```python
from build123d import *

# Parameters (mm, degrees)
SKETCH_1_W          = 45
SKETCH_1_H          = 70
SKETCH_1_R          = 2.25
SKETCH_1_R_2        = 2.5
SKETCH_1_R_3        = 1.75
SKETCH_1_R_4        = 0.9
SKETCH_1_R_5        = 0.75
EXTRUDE_1_DEPTH     = 1.5
SKETCH_2_R          = 0.6
CUT_EXTRUDE_1_DEPTH = 1.5


with BuildPart() as part:
    # Эскиз1 → Вытянуть1 (new body)
    with BuildSketch(Plane.XY):
        Rectangle(SKETCH_1_W, SKETCH_1_H)
        with Locations((-17.5, 30)):
            Circle(SKETCH_1_R, mode=Mode.SUBTRACT)
        with Locations(Location((17.5, 30, 0), (0, 0, 180))):
            Circle(SKETCH_1_R, mode=Mode.SUBTRACT)
        with Locations((17.5, -30)):
            Circle(SKETCH_1_R, mode=Mode.SUBTRACT)
        with Locations(Location((-17.5, -30, 0), (0, 0, 180))):
            Circle(SKETCH_1_R, mode=Mode.SUBTRACT)
        with Locations((0, -3)):
            Circle(SKETCH_1_R_2, mode=Mode.SUBTRACT)
        with Locations((-10.5, 7.5)):
            Circle(SKETCH_1_R_3, mode=Mode.SUBTRACT)
        with Locations((10.5, -13.5)):
            Circle(SKETCH_1_R_3, mode=Mode.SUBTRACT)
        with Locations((-5, 30)):
            Circle(SKETCH_1_R_4, mode=Mode.SUBTRACT)
        with Locations((0, 30)):
            Circle(SKETCH_1_R_4, mode=Mode.SUBTRACT)
        with Locations((5, 30)):
            Circle(SKETCH_1_R_4, mode=Mode.SUBTRACT)
        with Locations((-2.5, -30)):
            Circle(SKETCH_1_R_4, mode=Mode.SUBTRACT)
        with Locations((2.5, -30)):
            Circle(SKETCH_1_R_4, mode=Mode.SUBTRACT)
        with Locations((-4.5, -16.5)):
            Circle(SKETCH_1_R_5, mode=Mode.SUBTRACT)
        with Locations((-4.5, 10.5)):
            Circle(SKETCH_1_R_5, mode=Mode.SUBTRACT)
        with Locations(Location((4.5, -16.5, 0), (0, 0, 180))):
            Circle(SKETCH_1_R_5, mode=Mode.SUBTRACT)
        with Locations(Location((4.5, 10.5, 0), (0, 0, 180))):
            Circle(SKETCH_1_R_5, mode=Mode.SUBTRACT)
    extrude(amount=EXTRUDE_1_DEPTH)

    # Эскиз2 → Вырез-Вытянуть1 (cut)
    with BuildSketch(Plane.XY.offset(1.5)):
        with Locations((-17.5, -20.5)):
            Circle(SKETCH_2_R)
        with Locations((-17.5, 2.5)):
            Circle(SKETCH_2_R)
        with Locations(Location((17.5, 2.5, 0), (0, 0, 180))):
            Circle(SKETCH_2_R)
        with Locations(Location((17.5, -20.5, 0), (0, 0, 180))):
            Circle(SKETCH_2_R)
        with Locations((-7.5, -21.5)):
            Circle(SKETCH_2_R)
        with Locations((7.5, -21.5)):
            Circle(SKETCH_2_R)
        with Locations((-7.5, 15)):
            Circle(SKETCH_2_R)
        with Locations((7.5, 15)):
            Circle(SKETCH_2_R)
        with Locations((-10, 21.75)):
            Circle(SKETCH_2_R)
        with Locations(Location((10, 21.75, 0), (0, 0, 180))):
            Circle(SKETCH_2_R)
    extrude(amount=-CUT_EXTRUDE_1_DEPTH, mode=Mode.SUBTRACT)


solid = part.part
```
Geometry: final body of the model. Coordinates: model frame, mm. Round coordinates to 2 decimals unless told otherwise and drop trailing zeros. Write each loop counter-clockwise with the first axis right and the second up, starting at its lowest first coordinate (ties: lowest second). Pieces come first, ordered by that corner, then holes. Notation, with made-up numbers: M -22.75,39 L -2.75,39 A19 ccw -2.75,60 Z; hole C 50.25,-8 d9. An arc over 180 degrees is marked long. Answer in a Markdown table with one row per item. Add a question column.
(1) Ray query, L1, parallel to Y at x = 0, z = 0.45; L2, parallel to Y at x = 17.5, z = 0.45; L3, parallel to Y at x = -8, z = 1.25. Return the intervals inside material, ascending.
(2) Cut plane C-C, the plane x = 16. Return the cut outline in (y, z).
(3) Contact query for flat-ended pins moving along their axis: pin 1 (1.6 mm diameter, centred on x = 7.5, y = 15, fed in from +Z); pin 2 (2 mm diameter, centred on x = -10.5, y = 7.5, fed in from +Z) (3 decimals). Output: stop coordinate, or through.
(4) Draft query along X for faces 1 (the face through (5.05, 9.99, 0.74)), 2 (the face through (0, 0, 1.5)), 3 (the face through (22.5, 0, 1)). Return one class per face: pulls with the +X half, pulls with the -X half, needs draft (parallel to the pull), parting line crosses it, or undercut.
(5) Cut plane A-A, the plane y = 7.5. Return the cut outline in (x, z), then the cut area to 4 significant figures.
(6) Cut plane B-B, the plane z = 0.8. Give the number of separate pieces and of enclosed holes in the cut face, then the cut area to 3 significant figures.
Established:
| question | item | result |
|---|---|---|
| 1 | L1 | -35 to -5.5, -0.5 to 29.1, 30.9 to 35 |
| 1 | L2 | -35 to -32.25, -27.75 to -21.1, -19.9 to 1.9, 3.1 to 27.75, 32.25 to 35 |
| 1 | L3 | -35 to -21.83, -21.17 to 14.67, 15.33 to 35 |
| 2 | outline | M -35,0 L -31.68,0 L -31.68,1.5 L -35,1.5 Z; M -28.32,0 L 28.32,0 L 28.32,1.5 L -28.32,1.5 Z; M 31.68,0 L 35,0 L 35,1.5 L 31.68,1.5 Z |
| 3 | pin 1 | z = 1.5 |
| 3 | pin 2 | through |
| 4 | face 1 | undercut |
| 4 | face 2 | needs draft |
| 4 | face 3 | pulls with the +X half |
| 5 | outline | M -22.5,0 L -12.25,0 L -12.25,1.5 L -22.5,1.5 Z; M -8.75,0 L 22.5,0 L 22.5,1.5 L -8.75,1.5 Z |
| 5 | area | 62.25 mm² |
| 6 | separate pieces | 1 |
| 6 | enclosed holes | 26 |
| 6 | area | 3,020 mm² |
